Build history of the part. All positions in model axes, mm. Give positions to 0.01 mm unless a question says otherwise; leave off trailing zeros. Loops run counter-clockwise (first coordinate to the right, second up) from the corner with the lowest first, then second, coordinate; pieces in that order, holes last.
1) Band-saw the part on B-B on y = 0. List the corners of the cut face in (x, z), then the cut area to 3 significant figures.
2) Band-saw the part on A-A on z = 0. List the corners of the cut face in (x, y), then the cut area to 3 significant figures.
3) Wall check: line 1 (Z direction, x = 0.5, y = -8.75); line 2 (Y direction, x = 3.25, z = -0.25); line 3 (Z direction, x = 1.5, y = 3). Give the ranges that are in metal, low to high.
4) Flat gauge pins, fed straight in: P1, Ø2, axis at x = 5, z = 0, coming from the -Y side; P2, Ø6, axis at y = 6, z = 9, coming from the +X side; P3, Ø1.6, axis at x = 4, y = -1, coming from the -Z side. Where does each tip first touch, or does it go through?
```python
from build123d import *

# Parameters (mm, degrees)
BASPROSKE_W                 = 9
BASPROSKE_H                 = 14
TOOTHCUT_DEPTH              = 22.748563171
TEETHCUTS_COUNT             = 12
TEETHCUTS_ANGLE             = 330
BORSKE_R                    = 4
BORE_DEPTH                  = 50.0000508
DODANIE_WYCI_GNI_CIE1_START = 9
DODANIE_WYCI_GNI_CIE1_DEPTH = 9


with BuildPart() as part:
    # BasProSke → Base-Revolve (revolve)
    with BuildSketch(Plane(origin=(0, 0, 0), x_dir=(1, 0, 0), z_dir=(0, 1, 0)), mode=Mode.PRIVATE) as base_revolve_sk:
        with Locations((4.5, 7)):
            Rectangle(BASPROSKE_W, BASPROSKE_H)
    revolve(base_revolve_sk.sketch.rotate(Axis((-10, 0, 0), (1, 0, 0)), 180), axis=Axis((-10, 0, 0), (1, 0, 0)))

    # TooCutSke → ToothCut (cut, through all)
    with BuildSketch(Plane(origin=(0, 0, 0), x_dir=(0, 0, -1), z_dir=(1, 0, 0))):
        with BuildLine():
            ThreePointArc((1.111908866, 9.433698091), (0, 9.499), (-1.111908866, 9.433698091))
            ThreePointArc((-1.111908866, 9.433698091), (-1.651516138, 11.821129337), (-3.298149691, 13.632096456))
            ThreePointArc((-3.298149691, 13.632096456), (0, 14.0254), (3.298149691, 13.632096456))
            ThreePointArc((3.298149691, 13.632096456), (1.651516138, 11.821129337), (1.111908866, 9.433698091))
        make_face()
    toothcut = extrude(amount=TOOTHCUT_DEPTH, mode=Mode.SUBTRACT)

    # TeethCuts: ToothCut ×12 about axis
    teethcuts_axis = Axis((-10, 0, 0), (1, 0, 0))
    for i in range(1, TEETHCUTS_COUNT):
        add(toothcut.rotate(teethcuts_axis, i * TEETHCUTS_ANGLE / (TEETHCUTS_COUNT - 1)), mode=Mode.SUBTRACT)

    # BorSke → Bore (cut, symmetric)
    with BuildSketch(Plane(origin=(0, 0, 0), x_dir=(0, 0, -1), z_dir=(1, 0, 0))):
        with Locations(Location((0, 0, 0), (0, 0, 180))):
            Circle(BORSKE_R)
    extrude(amount=BORE_DEPTH, both=True, mode=Mode.SUBTRACT)

    # Szkic1 → Dodanie-wyciągnięcie1 (add)
    with BuildSketch(Plane(origin=(0, 0, 0), x_dir=(0, 0, -1), z_dir=(1, 0, 0)).offset(DODANIE_WYCI_GNI_CIE1_START)):
        with BuildLine():
            ThreePointArc((-3, 2.645751311), (-4, 0), (-3, -2.645751311))
            Line((-3, -2.645751311), (-3, 2.645751311))
        make_face()
    extrude(amount=-DODANIE_WYCI_GNI_CIE1_DEPTH)


solid = part.part
```
Findings below:
1. outline: (0, -9.5) - (9, -9.5) - (9, -4) - (0, -4) - close; (0, 3) - (9, 3) - (9, 9.5) - (0, 9.5) - close
1. area: 108 mm2
2. outline: (0, -9.5) - (9, -9.5) - (9, -4) - (0, -4) - close; (0, 4) - (9, 4) - (9, 9.5) - (0, 9.5) - close
2. area: 99.0 mm2
3. line 1: z = -10.02 to -6.52, -3.77 to 3.77, 6.52 to 10.02
3. line 2: y = -9.5 to -3.99, 3.99 to 9.5
3. line 3: z = -13.42 to -2.65, 2.65 to 13.42
4. P1: stops at y = -9.5
4. P2: stops at x = 9
4. P3: stops at z = -12.09
